For this review, take the finished solid that the model builds, in its own axes (mm). A direction names the side the tool comes from. Coordinates: 2 decimals unless noted, no trailing zeros. Write each loop counter-clockwise with the first axis right and the second up, starting at its lowest first coordinate (ties: lowest second). Pieces come first, ordered by that corner, then holes. Notation, with made-up numbers: (75.5, 44) -> (112.5, 44) arc R5 cw to (112.5, 53) -> close; hole circle Ø9 at (61.5, -5). An arc over 180 degrees is marked (long way). Put each result on its own line as item: value. Start each with the question number.
Item 1: To check wall thickness, follow L1, parallel to X at y = 4, z = 0.75; L2, parallel to X at y = 10.25, z = -4.5; L3, parallel to Z at x = -6, y = 11. State the ranges of each line that lie inside material, in increasing order.
Item 2: For faces 5 (the flat face through (0, 10, -3)), 6 (the flat face through (-3, 1, 0)), 7 (the flat face through (6, 1, -1.5)), 8 (the flat face through (-18.065, 9.5, -0.6)), list the 3-axis set-ups (+Z, -Z, +X, -X, +Y, -Y) from which the entire face can be reached by the end or side of a thin tool; tool diameter is ignored.
Item 3: The part is to be moulded in two halves that separate along Z. For faces 1 (the cylindrical face through (-17.6, 9.5, -3.8)), 2 (the flat face through (-16.74, 11.37, -8.79)), 3 (the cylindrical face through (3.84, 2.22, -0.38)), 4 (the flat face through (7, 4.5, 0)), say which applies: +Z half, -Z half, draft (parallel to the pull), parting line (faces both ways), or undercut.
Item 4: Consider section B-B on z = 0. Give the boundary of the cut face in (x, y).
Item 5: Consider section A-A on x = 8.5. Give the boundary of the cut face in (y, z), and give its area (3 significant figures).
Item 6: Consider section C-C on y = 12. Give the boundary of the cut face in (x, z).
Item 7: Consider section D-D on z = -7. Give the boundary of the cut face in (x, y), and give its area (3 significant figures).
Item 8: Insertion check: P1, Ø1.6, axis at x = 10, y = 1.5, coming from the -Z side; P2, Ø8, axis at x = 9, y = 2, coming from the +Z side; P3, Ø3, axis at x = -9, z = -4, coming from the +Y side; P4, Ø1, axis at y = 11.5, z = -6.5, coming from the -X side. Each pin has a flat end and moves straight along its axis. Give the tip position at first contact, or say it passes through.
```python
from build123d import *

# Parameters (mm, degrees)
SKETCH1_W             = 18
SKETCH1_H             = 3
BOSS_EXTRUDE1_DEPTH   = 9
BOSS_EXTRUDE2_DEPTH   = 4.8
CUT_EXTRUDE2_DEPTH    = 3.8
CUT_EXTRUDE3_DEPTH    = 6
CUT_EXTRUDE4_DEPTH    = 6.9
CUT_EXTRUDE5_DEPTH    = 4.5
SKETCH9_R             = 1
CUT_EXTRUDE6_DEPTH    = 4.5
SKETCH12_W            = 40.8
SKETCH12_H            = 4.8
CUT_EXTRUDE8_DEPTH    = 1.5
CHAMFER9_SIZE         = 7
CHAMFER9_SIZE2        = 5.873697418
CHAMFER9_PART_2_SIZE  = 7
CHAMFER9_PART_2_SIZE2 = 5.873697418


with BuildPart() as part:
    # Sketch1 → Boss-Extrude1 (new body)
    with BuildSketch(Plane(origin=(0, 0, 0), x_dir=(1, 0, 0), z_dir=(0, 1, 0))):
        with Locations((6, 0)):
            Rectangle(SKETCH1_W, SKETCH1_H)
    extrude(amount=BOSS_EXTRUDE1_DEPTH)

    # Sketch4 → Boss-Extrude2 (add)
    with BuildSketch(Plane(origin=(0, 9, 0), x_dir=(1, 0, 0), z_dir=(0, 1, 0))):
        Polygon((-16.265306784, 9.3), (16.265306784, 9.3), (20.4, 4.858031992), (20.4, -4.620102593), (-20.4, -4.620102593), (-20.4, 4.858031992), align=None)
    extrude(amount=BOSS_EXTRUDE2_DEPTH)

    # Sketch5 → Cut-Extrude2 (cut)
    with BuildSketch(Plane(origin=(0, 13.8, 0), x_dir=(1, 0, 0), z_dir=(0, 1, 0))):
        Polygon((16.513043846, 8.3), (-16.513043846, 8.3), (-19.4, 5.198496162), (-19.4, -3.620102593), (19.4, -3.620102593), (19.4, 5.198496162), align=None)
    extrude(amount=-CUT_EXTRUDE2_DEPTH, mode=Mode.SUBTRACT)

    # Sketch5<3> → Cut-Extrude3 (cut)
    with BuildSketch(Plane(origin=(0, 13.8, 0), x_dir=(1, 0, 0), z_dir=(0, 1, 0))):
        Polygon((20.4, -3.620102593), (19.4, -3.620102593), (-19.4, -3.620102593), (-20.4, -3.620102593), (-20.4, -4.620102593), (20.4, -4.620102593), align=None)
    extrude(amount=-CUT_EXTRUDE3_DEPTH, mode=Mode.SUBTRACT)

    # Sketch6 → Cut-Extrude4 (cut)
    with BuildSketch(Plane(origin=(0, 13.8, 0), x_dir=(1, 0, 0), z_dir=(0, 1, 0))):
        Polygon((-19.4, 5.198496162), (-19.4, 8.3), (-16.513043846, 8.3), align=None)
        Polygon((16.513043846, 8.3), (19.4, 5.198496162), (19.4, 8.3), align=None)
    extrude(amount=-CUT_EXTRUDE4_DEPTH, mode=Mode.SUBTRACT)

    # Sketch8 → Cut-Extrude5 (cut)
    with BuildSketch(Plane(origin=(0, 10, 0), x_dir=(1, 0, 0), z_dir=(0, 1, 0))):
        with BuildLine():
            Line((-17.065370438, 3.3), (-17.065370438, -4.992630539))
            ThreePointArc((-17.065370438, -4.992630539), (-17.565370438, -5.492630539), (-18.065370438, -4.992630539))
            Line((-18.065370438, -4.992630539), (-18.065370438, 3.3))
            ThreePointArc((-18.065370438, 3.3), (-17.565370438, 3.8), (-17.065370438, 3.3))
        make_face()
    extrude(amount=-CUT_EXTRUDE5_DEPTH, mode=Mode.SUBTRACT)

    # Sketch9 → Cut-Extrude6 (cut)
    with BuildSketch(Plane.XZ):
        with Locations((2.915469811, 0)):
            Circle(SKETCH9_R)
        with Locations((7.084530189, 0)):
            Circle(SKETCH9_R)
    extrude(amount=-CUT_EXTRUDE6_DEPTH, mode=Mode.SUBTRACT)

    # Sketch12 → Cut-Extrude8 (cut)
    with BuildSketch(Plane.XY.offset(3.620102593)):
        with Locations((0, 11.4)):
            Rectangle(SKETCH12_W, SKETCH12_H)
    extrude(amount=-CUT_EXTRUDE8_DEPTH, mode=Mode.SUBTRACT)

    # Chamfer9
    chamfer9_edges = [part.edges().sort_by_distance(p)[0] for p in [
        (6, 9, -1.5),
    ]]
    chamfer9_side = [part.faces().sort_by_distance(p)[0] for p in [
        (6, 4.5, -1.5),
    ]]
    chamfer(chamfer9_edges, length=CHAMFER9_SIZE, length2=CHAMFER9_SIZE2, reference=chamfer9_side[0])

    # Chamfer9 part 2
    chamfer9_part_2_edges = [part.edges().sort_by_distance(p)[0] for p in [
        (-3, 9, 0),
    ]]
    chamfer9_part_2_side = [part.faces().sort_by_distance(p)[0] for p in [
        (-3, 4.5, 0),
    ]]
    chamfer(chamfer9_part_2_edges, length=CHAMFER9_PART_2_SIZE, length2=CHAMFER9_PART_2_SIZE2, reference=chamfer9_part_2_side[0])


solid = part.part
```
Return value:
1. L1: -4.68 to 2.25, 3.58 to 6.42, 7.75 to 15
1. L2: -20.4 to -19.4, 19.4 to 20.4
1. L3: -9.3 to -8.3
2. face 5: +Z, +Y
2. face 6: +Z, -Z, -X, -Y
2. face 7: -Z, +X, -X, -Y
2. face 8: +Z, +Y, -Y
3. face 1: +Z half
3. face 2: -Z half
3. face 3: undercut
3. face 4: undercut
4. outline: (-20.4, 9) -> (-18.07, 9) -> (-18.07, 10) -> (-19.4, 10) -> (-19.4, 13.8) -> (-20.4, 13.8) -> close; (-17.07, 9) -> (-8.87, 9) -> (-3, 2) -> (-3, 0) -> (1.92, 0) -> (1.92, 4.5) -> (3.92, 4.5) -> (3.92, 0) -> (6.08, 0) -> (6.08, 4.5) -> (8.08, 4.5) -> (8.08, 0) -> (15, 0) -> (15, 9) -> (20.4, 9) -> (20.4, 13.8) -> (19.4, 13.8) -> (19.4, 10) -> (-17.07, 10) -> close
5. outline: (0, -1.5) -> (2, -1.5) -> (9, -7.37) -> (9, -9.3) -> (13.8, -9.3) -> (13.8, -8.3) -> (10, -8.3) -> (10, 2.12) -> (9, 2.12) -> (9, 1.5) -> (0, 1.5) -> close
5. area: 62.8 mm^2
6. outline: (-20.4, -4.86) -> (-19.4, -5.93) -> (-19.4, 2.12) -> (-20.4, 2.12) -> close; (-17.2, -8.3) -> (-16.27, -9.3) -> (16.27, -9.3) -> (17.2, -8.3) -> close; (19.4, -5.93) -> (20.4, -4.86) -> (20.4, 2.12) -> (19.4, 2.12) -> close
7. outline: (-17.72, 9) -> (-8.87, 9) -> (-8.5, 8.55) -> (15, 8.55) -> (15, 9) -> (17.72, 9) -> (17.72, 10) -> (-17.72, 10) -> close
7. area: 46.0 mm^2
8. P1: z = -1.75
8. P2: z = 1.5
8. P3: y = 10
8. P4: through
